Input: part model. Units: mm. Frame: model coordinates. A direction names the side the tool comes from. Give positions to 0.01 mm unless a question says otherwise; leave off trailing zeros. Write each loop counter-clockwise with the first axis right and the second up, starting at its lowest first coordinate (ties: lowest second). Pieces come first, ordered by that corner, then holes. Notation, with made-up numbers: (61, 83.5) - (93, 83.5) arc R19 ccw to (93, 100.5) - close; hole circle Ø1 at (-25, -3). An arc over 180 degrees is marked (long way). Use a Markdown table: item, result. Add a question column.
1. Material intervals for probe 1 along X at (y, z) = (2.95, -10); probe 2 along X at (y, z) = (2.9, -14.9); probe 3 along Z at (x, y) = (-20, 1.7), sorted ascending.
2. Set-up query: faces 1 (the cylindrical face through (-49.43, 2.46, 11.4)), 2 (the flat face through (0, 2, 2)). Return all of +Z, -Z, +X, -X, +Y, -Y with unobstructed straight access to the full face (end or side cutting, diameter ignored); none if empty.
3. Section query B-B, the plane y = 3.4. Count the separate pieces of the cut face and the enclosed holes in it, plus the area to 3 significant figures.
4. Pin query (flat end, axial travel): pin 1 (2.5 mm diameter, centred on x = 10, z = -10, fed in from +Y). Return the tip coordinate at first contact, or that it passes through.
5. Mould query, pull axis X, two halves, no side actions, for faces 3 (the cylindrical face through (-9.625, 2.465, 7.285)), 4 (the flat face through (-1, 0, -6)), 5 (the flat face through (-50, 2, -6)). Classes: released by +X, released by -X, zero draft, split by the parting line, or undercut.
6. Section query A-A, the plane z = -10. Return loops of the section in (x, y).
```python
from build123d import *

# Parameters (mm, degrees)
SKETCH1_R           = 1.3
SKETCH1_R_2         = 2.05
SKETCH1_R_3         = 1.55
BOSS_EXTRUDE1_DEPTH = 5


with BuildPart() as part:
    # Sketch1 → Boss-Extrude1 (new body)
    with BuildSketch(Plane(origin=(0, 0, 0), x_dir=(1, 0, 0), z_dir=(0, 1, 0))):
        with BuildLine():
            Line((-48, -12), (48, -12))
            ThreePointArc((48, -12), (49.414213562, -11.414213562), (50, -10))
            Line((50, -10), (50, 22))
            ThreePointArc((50, 22), (49.414213562, 23.414213562), (48, 24))
            Line((48, 24), (-48, 24))
            ThreePointArc((-48, 24), (-49.414213562, 23.414213562), (-50, 22))
            Line((-50, 22), (-50, -10))
            ThreePointArc((-50, -10), (-49.414213562, -11.414213562), (-48, -12))
        make_face()
        with Locations(Location((0, 7.6, 0), (0, 0, 270))):
            Circle(SKETCH1_R, mode=Mode.SUBTRACT)
        with Locations(Location((6.581793069, -3.8, 0), (0, 0, 270))):
            Circle(SKETCH1_R, mode=Mode.SUBTRACT)
        with Locations(Location((-6.581793069, -3.8, 0), (0, 0, 90))):
            Circle(SKETCH1_R, mode=Mode.SUBTRACT)
        with Locations(Location((44, 14.9, 0), (0, 0, 270))):
            Circle(SKETCH1_R_2, mode=Mode.SUBTRACT)
        with Locations(Location((20, 14.9, 0), (0, 0, 270))):
            Circle(SKETCH1_R_2, mode=Mode.SUBTRACT)
        with Locations(Location((44, -3.1, 0), (0, 0, 270))):
            Circle(SKETCH1_R_2, mode=Mode.SUBTRACT)
        with Locations(Location((20, -3.1, 0), (0, 0, 270))):
            Circle(SKETCH1_R_2, mode=Mode.SUBTRACT)
        with Locations(Location((-44, -3.1, 0), (0, 0, 90))):
            Circle(SKETCH1_R_2, mode=Mode.SUBTRACT)
        with Locations(Location((-20, -3.1, 0), (0, 0, 90))):
            Circle(SKETCH1_R_2, mode=Mode.SUBTRACT)
        with Locations(Location((-20, 14.9, 0), (0, 0, 90))):
            Circle(SKETCH1_R_2, mode=Mode.SUBTRACT)
        with Locations(Location((-44, 14.9, 0), (0, 0, 90))):
            Circle(SKETCH1_R_2, mode=Mode.SUBTRACT)
        with Locations(Location((11, -8, 0), (0, 0, 270))):
            Circle(SKETCH1_R_3, mode=Mode.SUBTRACT)
        with Locations(Location((10, 10, 0), (0, 0, 270))):
            Circle(SKETCH1_R_3, mode=Mode.SUBTRACT)
        with Locations(Location((-11, -8, 0), (0, 0, 90))):
            Circle(SKETCH1_R_3, mode=Mode.SUBTRACT)
        with Locations(Location((-10, 10, 0), (0, 0, 90))):
            Circle(SKETCH1_R_3, mode=Mode.SUBTRACT)
        with BuildLine():
            Line((2, 4), (-2, 4))
            ThreePointArc((-2, 4), (-5, 1), (-2, -2))
            Line((-2, -2), (2, -2))
            ThreePointArc((2, -2), (5, 1), (2, 4))
        make_face(mode=Mode.SUBTRACT)
    extrude(amount=BOSS_EXTRUDE1_DEPTH)


solid = part.part
```
Result sheet:
| question | item | result |
|---|---|---|
| 1 | probe 1 | x = -50 to -11.55, -8.45 to 8.45, 11.55 to 50 |
| 1 | probe 2 | x = -50 to -46.05, -41.95 to -22.05, -17.95 to 17.95, 22.05 to 41.95, 46.05 to 50 |
| 1 | probe 3 | z = -24 to -16.95, -12.85 to 1.05, 5.15 to 12 |
| 2 | face 1 | +Z, -X, +Y, -Y |
| 2 | face 2 | +Y, -Y |
| 3 | separate pieces | 1 |
| 3 | enclosed holes | 16 |
| 3 | area | 3,390 mm² |
| 4 | pin 1 | passes through |
| 5 | face 3 | undercut |
| 5 | face 4 | zero draft |
| 5 | face 5 | released by -X |
| 6 | outline | (-50, 0) - (-11.55, 0) - (-11.55, 5) - (-50, 5) - close; (-8.45, 0) - (8.45, 0) - (8.45, 5) - (-8.45, 5) - close; (11.55, 0) - (50, 0) - (50, 5) - (11.55, 5) - close |
